Here's how the part is built. I have some questions about the finished solid (model axes, mm). Face numbers are marked on the shaded views. A direction names the side the tool comes from. Give positions to 0.01 mm unless a question says otherwise; leave off trailing zeros. Loops run counter-clockwise (first coordinate to the right, second up) from the corner with the lowest first, then second, coordinate; pieces in that order, holes last.
Q1. I'm going to push flat-ended pins straight in: P1, Ø10, axis at y = 313.5, z = 31.5, coming from the -X side; P2, Ø6, axis at y = 310, z = -13, coming from the +X side; P3, Ø18, axis at x = 236, z = -162, coming from the +Y side. Where does each tip first touch, or does it pass through?
Q2. For the marked faces 4 and 5, which set-ups out of +Z, -Z, +X, -X, +Y, -Y let a thin tool reach every point of the face, with its end or its side?
Q3. Suppose I cut it at B-B (x = 46.5). List the corners of the cut face in (y, z) for me, and give its area (3 significant figures).
Q4. Suppose I cut it at A-A (y = 150). List the corners of the cut face in (x, z) for me.
Q5. Suppose I cut it at C-C (z = 0). List the corners of the cut face in (x, y) for me, and give its area (3 significant figures).
Q6. I need wall thicknesses on probe 1 along Z at (x, y) = (225, 165); probe 2 along Z at (x, y) = (112, 150); probe 3 along X at (y, z) = (205, -35). Which ranges of each line are inside material? Lowest first, please.
Q7. Thinking about a two-plate mould opening in Z: for the marked faces 1, 2 and 3, which applies, pulls with the +Z half, pulls with the -Z half, needs draft (parallel to the pull), parting line crosses it, or undercut?
Q8. Suppose I cut it at D-D (x = 225). List the corners of the cut face in (y, z) for me, and give its area (3 significant figures).
```python
from build123d import *

# Parameters (mm, degrees)
SKETCH1_W               = 850
SKETCH1_H               = 700
SKETCH1_R               = 105
BOSS_EXTRUDE1_DEPTH     = 300
SKETCH2_W               = 718.724675112
SKETCH2_H               = 607.354725455
BOSS_EXTRUDE2_DEPTH     = 100
SKETCH3_R               = 30
BOSS_EXTRUDE3_DEPTH     = 10
CUT_EXTRUDE1_START      = -325
SKETCH4_R               = 141
CUT_EXTRUDE1_DEPTH      = 200
CUT_EXTRUDE2_DEPTH      = 220
CUT_EXTRUDE2_DEPTH_BACK = 20
SKETCH5_R               = 50
SKETCH6_W               = 200
SKETCH6_H               = 200
BOSS_EXTRUDE4_DEPTH     = 20


with BuildPart() as part:
    # Sketch1 → Boss-Extrude1 (new body)
    with BuildSketch(Plane(origin=(0, 0, 0), x_dir=(1, 0, 0), z_dir=(0, 1, 0))):
        Rectangle(SKETCH1_W, SKETCH1_H)
        with Locations(Location((-225, 150, 0), (0, 0, 270))):
            Circle(SKETCH1_R, mode=Mode.SUBTRACT)
        with Locations(Location((225, 150, 0), (0, 0, 270))):
            Circle(SKETCH1_R, mode=Mode.SUBTRACT)
        with Locations(Location((-225, -150, 0), (0, 0, 270))):
            Circle(SKETCH1_R, mode=Mode.SUBTRACT)
        with Locations(Location((225, -150, 0), (0, 0, 270))):
            Circle(SKETCH1_R, mode=Mode.SUBTRACT)
    extrude(amount=BOSS_EXTRUDE1_DEPTH)

    # Sketch2 → Boss-Extrude2 (add)
    with BuildSketch(Plane.XZ):
        with Locations((3.884998244, -5.179997659)):
            Rectangle(SKETCH2_W, SKETCH2_H)
    extrude(amount=-BOSS_EXTRUDE2_DEPTH)

    # Sketch3 → Boss-Extrude3 (add)
    with BuildSketch(Plane(origin=(0, 100, 0), x_dir=(1, 0, 0), z_dir=(0, 1, 0))):
        with Locations(Location((-225, 150, 0), (0, 0, 90))):
            Circle(SKETCH3_R)
        with Locations(Location((225, 150, 0), (0, 0, 90))):
            Circle(SKETCH3_R)
        with Locations(Location((225, -150, 0), (0, 0, 90))):
            Circle(SKETCH3_R)
        with Locations(Location((-225, -150, 0), (0, 0, 90))):
            Circle(SKETCH3_R)
    extrude(amount=BOSS_EXTRUDE3_DEPTH)

    # Sketch4 → Cut-Extrude1 (cut)
    with BuildSketch(Plane.ZY.offset(425).offset(CUT_EXTRUDE1_START)):
        with Locations((0, 150)):
            Circle(SKETCH4_R)
    extrude(amount=-CUT_EXTRUDE1_DEPTH, mode=Mode.SUBTRACT)

    # Sketch5 → Cut-Extrude2 (cut, two sides: drawn at the far end of the back side and taken through both)
    with BuildSketch(Plane.ZY.offset(-100).offset(-CUT_EXTRUDE2_DEPTH_BACK)):
        with Locations((0, 150)):
            Circle(SKETCH5_R)
    extrude(amount=CUT_EXTRUDE2_DEPTH + CUT_EXTRUDE2_DEPTH_BACK, mode=Mode.SUBTRACT)

    # Sketch6 → Boss-Extrude4 (add)
    with BuildSketch(Plane(origin=(0, 300, 0), x_dir=(1, 0, 0), z_dir=(0, 1, 0))):
        Rectangle(SKETCH6_W, SKETCH6_H)
    extrude(amount=BOSS_EXTRUDE4_DEPTH)


solid = part.part
```
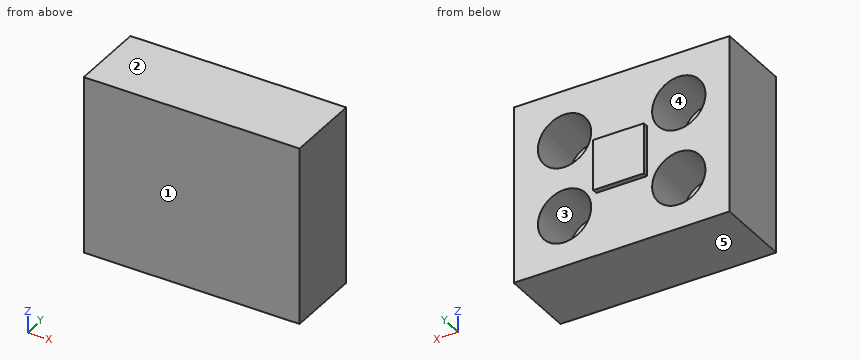
Solutions:
1. P1: stops at x = -100
1. P2: stops at x = 100
1. P3: stops at y = 110
2. face 4: +Y
2. face 5: -Z, +X, -X, +Y, -Y
3. outline: (0, -350) - (300, -350) - (300, -100) - (320, -100) - (320, 100) - (300, 100) - (300, 350) - (0, 350) - close; hole circle Ø282 at (150, 0)
3. area: 152,000 mm2
4. outline: (-425, -350) - (425, -350) - (425, 350) - (-425, 350) - close; hole circle Ø210 at (-225, -150); hole circle Ø210 at (-225, 150); hole (-120, -50) - (-100, -50) - (-100, -141) - (100, -141) - (100, -50) - (120, -50) - (120, 50) - (100, 50) - (100, 141) - (-100, 141) - (-100, 50) - (-120, 50) - close; hole circle Ø210 at (225, -150); hole circle Ø210 at (225, 150)
5. outline: (-425, 0) - (425, 0) - (425, 300) - (100, 300) - (100, 320) - (-100, 320) - (-100, 300) - (-425, 300) - close; hole (-120, 100) - (-100, 100) - (-100, 9) - (100, 9) - (100, 100) - (120, 100) - (120, 200) - (100, 200) - (100, 291) - (-100, 291) - (-100, 200) - (-120, 200) - close
5. area: 199,000 mm2
6. probe 1: z = -350 to -255, -45 to 45, 255 to 350
6. probe 2: z = -350 to -50, 50 to 350
6. probe 3: x = -425 to -100, 100 to 425
7. face 1: needs draft
7. face 2: pulls with the +Z half
7. face 3: undercut
8. outline: (0, -350) - (300, -350) - (300, -255) - (100, -255) - (100, -180) - (110, -180) - (110, -120) - (100, -120) - (100, -45) - (300, -45) - (300, 45) - (100, 45) - (100, 120) - (110, 120) - (110, 180) - (100, 180) - (100, 255) - (300, 255) - (300, 350) - (0, 350) - close
8. area: 127,000 mm2
